```python
from build123d import *

# Parameters (mm, degrees)
F0_R     = 11.25
F1_DEPTH = 37
F2_R     = 9.75
F3_DEPTH = 35
F4_R     = 10.3
F5_DEPTH = 5
F6_SIZE  = 0.1
F7_SIZE  = 0.2


with BuildPart() as f1:
    # F0 (on Top) → F1 (new body)
    with BuildSketch(Plane.XY):
        Circle(F0_R)
    extrude(amount=F1_DEPTH)

    # F2 (on face) → F3 (cut)
    with BuildSketch(Plane.XY.offset(37)):
        Circle(F2_R)
    extrude(amount=-F3_DEPTH, mode=Mode.SUBTRACT)

    # F4 (on face) → F5 (cut)
    with BuildSketch(Plane.XY.offset(37)):
        Circle(F4_R)
    extrude(amount=-F5_DEPTH, mode=Mode.SUBTRACT)

    # F6
    f6_edges = [f1.edges().sort_by_distance(p)[0] for p in [
        (-10.3, 0, 37),
        (-11.25, 0, 37),
        (-9.75, 0, 32),
    ]]
    chamfer(f6_edges, length=F6_SIZE)

    # F7
    f7_edges = [f1.edges().sort_by_distance(p)[0] for p in [
        (-11.25, 0, 0),
    ]]
    chamfer(f7_edges, length=F7_SIZE)


solid = f1.part
```
Source: CAD feature listing. Evaluate the final solid. Frame: model axes, mm. Coordinates: 2 decimals unless noted, no trailing zeros. Loops run counter-clockwise (first coordinate to the right, second up) from the corner with the lowest first, then second, coordinate; pieces in that order, holes last. Notation, with made-up numbers: (31.25, 62) -> (84.25, 62) arc R21 cw to (84.25, 69) -> close; hole circle Ø8 at (-0.5, -19.75). An arc over 180 degrees is marked (long way). One line per item, written item: value. Start each with the question number.
Q1. Contact query for flat-ended pins moving along their axis: P1, Ø6, axis at x = -4.5, y = -1, coming from the +Z side; P2, Ø3, axis at y = 7, z = 19.5, coming from the -X side; P3, Ø4, axis at y = 5.5, z = 22.5, coming from the -X side. Output: stop coordinate, or through.
Q2. Line query: line 1 along Y through (x, z) = (0, 23.5); line 2 along Y through (x, z) = (0, 33.45); line 3 along Z through (x, y) = (2, -9). Output: solid intervals per line, ascending.
Q3. Section query A-A, the plane x = 0. Return the cut outline in (y, z).
Q4. Mould query, pull axis X, two halves, no side actions, for faces 1 (the face through (0, 0, 0)), 2 (the face through (5.19, -9.98, 18.29)), 3 (the face through (1, -10, 32)). Classes: pulls with the +X half, pulls with the -X half, needs draft (parallel to the pull), parting line crosses it, or undercut.
Q5. Section query C-C, the plane z = 12. Return the cut outline in (x, y).
Results:
1. P1: z = 2
1. P2: x = -9.81
1. P3: x = -10.69
2. line 1: -11.25 to -9.75, 9.75 to 11.25
2. line 2: -11.25 to -10.3, 10.3 to 11.25
2. line 3: 0 to 2
3. outline: (-11.25, 0.2) -> (-11.05, 0) -> (11.05, 0) -> (11.25, 0.2) -> (11.25, 36.9) -> (11.15, 37) -> (10.4, 37) -> (10.3, 36.9) -> (10.3, 32) -> (9.85, 32) -> (9.75, 31.9) -> (9.75, 2) -> (-9.75, 2) -> (-9.75, 31.9) -> (-9.85, 32) -> (-10.3, 32) -> (-10.3, 36.9) -> (-10.4, 37) -> (-11.15, 37) -> (-11.25, 36.9) -> close
4. face 1: needs draft
4. face 2: parting line crosses it
4. face 3: undercut
5. outline: circle Ø22.5 at (0, 0); hole circle Ø19.5 at (0, 0)
